The listing builds one solid part. Answer for the finished solid, in the listing's coordinates (mm). Coordinates: 2 decimals unless noted, no trailing zeros. Write each loop counter-clockwise with the first axis right and the second up, starting at its lowest first coordinate (ties: lowest second). Pieces come first, ordered by that corner, then holes. Notation, with made-up numbers: M 86,45.5 L 141,45.5 A22 ccw 141,77.5 Z; hole C 22.5,-20.75 d5. An arc over 180 degrees is marked long. Answer as CSV lines item,"result". Start each with the question number.
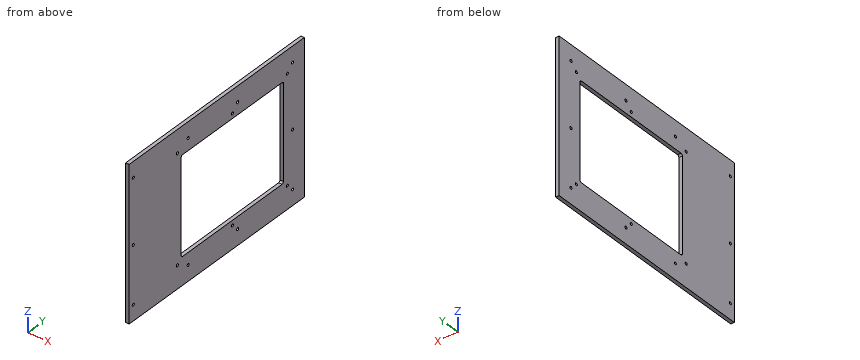
```python
from build123d import *

# Parameters (mm, degrees)
SKETCH1_W           = 542.925
SKETCH1_H           = 809.625
BOSS_EXTRUDE1_DEPTH = 12.7
SKETCH2_R           = 4.7625
CUT_EXTRUDE1_DEPTH  = 12.7
SKETCH3_R           = 4.7625
CUT_EXTRUDE2_DEPTH  = 12.7
SKETCH6_R           = 4.7625
CUT_EXTRUDE4_DEPTH  = 12.7
SKETCH7_R           = 4.7625
CUT_EXTRUDE5_DEPTH  = 12.7
SKETCH9_W           = 346.075
SKETCH9_H           = 473.075
CUT_EXTRUDE6_DEPTH  = 12.7
FILLET1_R           = 6.35


with BuildPart() as part:
    # Sketch1 → Boss-Extrude1 (new body)
    with BuildSketch(Plane(origin=(0, 0, 0), x_dir=(0, 0, -1), z_dir=(1, 0, 0))):
        Rectangle(SKETCH1_W, SKETCH1_H)
    extrude(amount=BOSS_EXTRUDE1_DEPTH)

    # Sketch2 → Cut-Extrude1 (cut)
    with BuildSketch(Plane(origin=(12.7, 0, 0), x_dir=(0, 0, -1), z_dir=(1, 0, 0))):
        with Locations((-215.9, 350.52)):
            Circle(SKETCH2_R)
        with Locations((215.9, 350.52)):
            Circle(SKETCH2_R)
        with Locations((-215.9, -386.08)):
            Circle(SKETCH2_R)
        with Locations((215.9, -386.08)):
            Circle(SKETCH2_R)
    extrude(amount=-CUT_EXTRUDE1_DEPTH, mode=Mode.SUBTRACT)

    # Sketch3 → Cut-Extrude2 (cut)
    with BuildSketch(Plane(origin=(12.7, 0, 0), x_dir=(0, 0, -1), z_dir=(1, 0, 0))):
        with Locations((-215.9, 96.52)):
            Circle(SKETCH3_R)
        with Locations((-215.9, -132.08)):
            Circle(SKETCH3_R)
        with Locations((12.7, 350.52)):
            Circle(SKETCH3_R)
        with Locations((12.7, -386.08)):
            Circle(SKETCH3_R)
        with Locations(Location((215.9, -132.08, 0), (0, 0, 180))):
            Circle(SKETCH3_R)
        with Locations(Location((215.9, 96.52, 0), (0, 0, 180))):
            Circle(SKETCH3_R)
    extrude(amount=-CUT_EXTRUDE2_DEPTH, mode=Mode.SUBTRACT)

    # Sketch6 → Cut-Extrude4 (cut)
    with BuildSketch(Plane.ZY):
        with Locations((-190.5, 325.91375)):
            Circle(SKETCH6_R)
        with Locations((190.5, 325.91375)):
            Circle(SKETCH6_R)
        with Locations((-190.5, -182.08625)):
            Circle(SKETCH6_R)
        with Locations((190.5, -182.08625)):
            Circle(SKETCH6_R)
    extrude(amount=-CUT_EXTRUDE4_DEPTH, mode=Mode.SUBTRACT)

    # Sketch7 → Cut-Extrude5 (cut)
    with BuildSketch(Plane.ZY):
        with Locations((-190.5, 71.91375)):
            Circle(SKETCH7_R)
        with Locations((190.5, 71.91375)):
            Circle(SKETCH7_R)
    extrude(amount=-CUT_EXTRUDE5_DEPTH, mode=Mode.SUBTRACT)

    # Sketch9 → Cut-Extrude6 (cut)
    with BuildSketch(Plane(origin=(12.7, 0, 0), x_dir=(0, 0, -1), z_dir=(1, 0, 0))):
        with Locations((0, 71.91375)):
            Rectangle(SKETCH9_W, SKETCH9_H)
    extrude(amount=-CUT_EXTRUDE6_DEPTH, mode=Mode.SUBTRACT)

    # Fillet1
    fillet1_edges = [part.edges().sort_by_distance(p)[0] for p in [
        (6.35, -164.62375, -173.0375),
        (6.35, -164.62375, 173.0375),
        (6.35, 308.45125, 173.0375),
        (6.35, 308.45125, -173.0375),
    ]]
    fillet(fillet1_edges, radius=FILLET1_R)


solid = part.part
```
1) This flat-tipped pin is pushed along its axis until it touches: P1, Ø12.5, axis at y = -386.08, z = -12.7, coming from the +X side. Where does it stop, or does it pass through?
2) The part is cut by section A-A (z = 154.5). Determine the outline of the cut face in (x, y).
3) The part is cut by section C-C (x = 3). Count the separate pieces of the cut face and the enclosed holes in it, then the cut area to 3 significant figures.
4) The part is cut by section B-B (y = 34). Determine the outline of the cut face in (x, z), then the cut area to 3 significant figures.
5) Find the intervals of material crossed by line 1 (Z direction, x = 9.25, y = 350.52); line 2 (Y direction, x = 9.75, z = 215.9); line 3 (Y direction, x = 8.25, z = -190.5), in increasing order. Write a range as from..to.
Completed:
1,P1,"x = 12.7"
2,outline,"M 0,-404.81 L 12.7,-404.81 L 12.7,-164.62 L 0,-164.62 Z; M 0,308.45 L 12.7,308.45 L 12.7,404.81 L 0,404.81 Z"
3,separate pieces,"1"
3,enclosed holes,"17"
3,area,"275,000 mm²"
4,outline,"M 0,-271.46 L 12.7,-271.46 L 12.7,-173.04 L 0,-173.04 Z; M 0,173.04 L 12.7,173.04 L 12.7,271.46 L 0,271.46 Z"
4,area,"2,500 mm²"
5,line 1,"-271.46..-220.66, -211.14..-17.46, -7.94..211.14, 220.66..271.46"
5,line 2,"-404.81..-390.84, -381.32..-136.84, -127.32..91.76, 101.28..345.76, 355.28..404.81"
5,line 3,"-404.81..-186.85, -177.32..67.15, 76.68..321.15, 330.68..404.81"
